Can you work these out from the model? Positions are in its coordinate system, mm. A direction names the side the tool comes from. Give positions to 0.01 mm unless a question says otherwise; leave off trailing zeros. Loops run counter-clockwise (first coordinate to the right, second up) from the corner with the lowest first, then second, coordinate; pieces in that order, holes last. Notation, with made-up numbers: M 86,5 L 143,5 A7 cw 143,12 Z; hole C 35.5,36.25 d3. An arc over 180 degrees is marked long. Answer as a JSON object with one key per item and string values.
```python
from build123d import *

# Parameters (mm, degrees)
SKETCH003_W   = 7.4
SKETCH003_H   = 6
PAD003_DEPTH  = 6.25
SKETCH004_R   = 1.5
PAD004_DEPTH  = 3.25
CHAMFER_ANGLE = 85.55
CHAMFER_SIZE  = 0.25


with BuildPart() as part:
    # Sketch003 → Pad003 (new body)
    with BuildSketch(Plane.YZ):
        with Locations((-4.647178, 8.71105)):
            Rectangle(SKETCH003_W, SKETCH003_H)
    extrude(amount=PAD003_DEPTH)

    # Sketch004 (on Face6 of Pad003) → Pad004 (join)
    with BuildSketch(Plane.YZ.offset(6.25)):
        with Locations((-4.647178, 8.71105)):
            Circle(SKETCH004_R)
    extrude(amount=PAD004_DEPTH)

    # Chamfer
    chamfer_edges = [part.edges().sort_by_distance(p)[0] for p in [
        (6.25, -6.147178, 8.71105),
    ]]
    chamfer_side = part.faces().sort_by_distance((6.25, -8.25191, 8.71105))[0]
    chamfer(chamfer_edges, length=CHAMFER_SIZE, angle=CHAMFER_ANGLE, reference=chamfer_side)


solid = part.part
```
1) Please list where these lines run through material, in increasing order: line 1 along X through (y, z) = (-7.5, 9.85); line 2 along Y through (x, z) = (8.5, 10.1); line 3 along Y through (x, z) = (6.5, 10.15). Write a range as from..to.
Answer list:
{"line 1": "0..6.25", "line 2": "-5.39..-3.9", "line 3": "-5.61..-3.69"}
2) Suppose I cut it at B-B, the plane z = 6.6. Write out the boundary of the cut face in (x, y).
Answer list:
{"outline": "M 0,-8.35 L 6.25,-8.35 L 6.25,-0.95 L 0,-0.95 Z"}
3) Suppose I cut it at A-A, the plane y = -2.5. Write out the boundary of the cut face in (x, z).
Answer list:
{"outline": "M 0,5.71 L 6.25,5.71 L 6.25,11.71 L 0,11.71 Z"}
4) For faces 1 (the flat face through (6.25, -4.7, 6.8)), 2 (the flat face through (3, -8.347, 9)), which set-ups out of +Z, -Z, +X, -X, +Y, -Y let a thin tool reach every point of the face, with its end or its side?
Answer list:
{"face 1": "+X", "face 2": "+Z, -Z, +X, -X, -Y"}
